Autodesk Inventor part; units mm, degrees
ref_plane "YZ Plane" through (0, 0, 0) normal (1, 0, 0) x (0, 1, 0)
ref_plane "XZ Plane" through (0, 0, 0) normal (0, 1, 0) x (-1, 0, 0)
ref_plane "XY Plane" through (0, 0, 0) normal (0, 0, 1) x (1, 0, 0)
sketch "Эскиз1" plane through (0, 0, 0) normal (0, 0, 1) x (1, 0, 0)
  line L0 (-15.776, 404) -> (-10, 404)
  line L1 (0, 404) -> (-10, 404)
  line L2 (0, 404) -> (0, 408)
  line L3 (-10, 408) -> (0, 408)
  line L4 (-10, 404) -> (-10, 408)
  line L5 (20, 404) -> (10, 404)
  line L6 (20, 404) -> (20, 408)
  line L7 (10, 408) -> (20, 408)
  line L8 (10, 404) -> (10, 408)
  line L9 (0, 404) -> (10, 404)
  line L10 (20, 404) -> (30, 404)
  line L11 (40, 404) -> (30, 404)
  line L12 (40, 404) -> (40, 408)
  line L13 (30, 408) -> (40, 408)
  line L14 (30, 404) -> (30, 408)
  line L15 (40, 404) -> (50, 404)
  line L16 (60, 404) -> (50, 404)
  line L17 (60, 404) -> (60, 408)
  line L18 (50, 408) -> (60, 408)
  line L19 (50, 404) -> (50, 408)
  line L20 (60, 404) -> (70, 404)
  line L21 (70, 404) -> (80, 404)
  line L22 (80, 404) -> (80, 408)
  line L23 (70, 408) -> (80, 408)
  line L24 (70, 404) -> (70, 408)
  line L25 (80, 404) -> (90.6418, 404)
  line L26 (-15.776, 4) -> (-10, 4)
  line L27 (0, 0) -> (-10, 0)
  line L28 (0, 0) -> (0, 4)
  line L29 (-10, 4) -> (0, 4)
  line L30 (-10, 0) -> (-10, 4)
  line L31 (0, 4) -> (10, 4)
  line L32 (20, 0) -> (10, 0)
  line L33 (20, 0) -> (20, 4)
  line L34 (10, 4) -> (20, 4)
  line L35 (10, 0) -> (10, 4)
  line L36 (20, 4) -> (30, 4)
  line L37 (40, 0) -> (30, 0)
  line L38 (40, 0) -> (40, 4)
  line L39 (30, 4) -> (40, 4)
  line L40 (30, 0) -> (30, 4)
  line L41 (60, 0) -> (50, 0)
  line L42 (60, 0) -> (60, 4)
  line L43 (50, 4) -> (60, 4)
  line L44 (50, 0) -> (50, 4)
  line L45 (40, 4) -> (50, 4)
  line L46 (60, 4) -> (70, 4)
  line L47 (70, 0) -> (80, 0)
  line L48 (80, 0) -> (80, 4)
  line L49 (70, 4) -> (80, 4)
  line L50 (70, 0) -> (70, 4)
  line L51 (80, 4) -> (90.6418, 4)
  line L52 (90.6418, 4) -> (90.6418, 404)
  line L53 (-15.776, 404) -> (-10, 404)
  line L54 (-15.776, 4) -> (-15.776, 404)
extrude "Выдавливание1" add sketch "Эскиз1" along normal blind 4
properties part number "верх"
Source: CAD feature listing. Evaluate the final solid. Frame: model axes, mm. Coordinates: 2 decimals unless noted, no trailing zeros. Loops run counter-clockwise (first coordinate to the right, second up) from the corner with the lowest first, then second, coordinate; pieces in that order, holes last. Notation, with made-up numbers: (-32.75, -15) - (7.25, -15) arc R22 ccw to (7.25, 3) - close; hole circle Ø4 at (33, 54). An arc over 180 degrees is marked (long way). Return JSON: item names as keys, results as strings.
Q1. Contact query for flat-ended pins moving along their axis: P1, Ø2, axis at y = 406.5, z = 2.5, coming from the +X side; P2, Ø1.2, axis at x = 22.5, z = 1.5, coming from the -Y side; P3, Ø1.2, axis at x = 25.5, z = 3, coming from the +Y side. Output: stop coordinate, or through.
Results:
{"P1": "x = 80", "P2": "y = 4", "P3": "y = 404"}
Q2. Material intervals for line 1 along Y through (x, z) = (-11, 3.15), sorted ascending.
Results:
{"line 1": "4 to 404"}
Q3. Section A-A, the plane x = 46.5. Return loops of the section in (y, z), plus the area to 3 significant figures.
Results:
{"outline": "(4, 0) - (404, 0) - (404, 4) - (4, 4) - close", "area": "1,600 mm2"}
